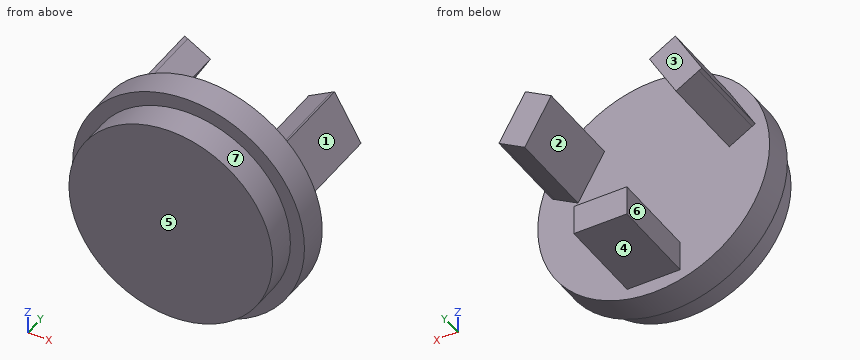
from build123d import *

# Parameters (mm, degrees)
ESQUISSE2_R        = 61.5
BOSS_EXTRU_1_DEPTH = 18
ESQUISSE3_R        = 70
BOSS_EXTRU_2_DEPTH = 18
BOSS_EXTRU_3_DEPTH = 54


with BuildPart() as part:
    # Esquisse2 → Boss.-Extru.1 (new body)
    with BuildSketch(Plane(origin=(0, 0, 0), x_dir=(1, 0, 0), z_dir=(0, 1, 0))):
        with Locations(Location((50.887518325, 23.784383565, 0), (0, 0, 270))):
            Circle(ESQUISSE2_R)
    extrude(amount=BOSS_EXTRU_1_DEPTH)

    # Esquisse3 → Boss.-Extru.2 (add)
    with BuildSketch(Plane(origin=(0, 18, 0), x_dir=(1, 0, 0), z_dir=(0, 1, 0))):
        with Locations(Location((50.887518325, 23.784383565, 0), (0, 0, 270))):
            Circle(ESQUISSE3_R)
    extrude(amount=BOSS_EXTRU_2_DEPTH)

    # Esquisse4 → Boss.-Extru.3 (add)
    with BuildSketch(Plane(origin=(0, 36, 0), x_dir=(1, 0, 0), z_dir=(0, 1, 0))):
        with BuildLine():
            ThreePointArc((-2.373044008, -6.965616435), (2.122342369, -13.688374727), (7.460993068, -19.763141096))
            Line((7.460993068, -19.763141096), (21.215413261, -11.822022896))
            Line((21.215413261, -11.822022896), (13.215413261, 2.034383565))
            Line((13.215413261, 2.034383565), (5.215413261, 15.890790026))
            Line((5.215413261, 15.890790026), (-8.539006932, 7.949671825))
            ThreePointArc((-8.539006932, 7.949671825), (-5.947430283, 0.288881513), (-2.373044008, -6.965616435))
        make_face()
        with BuildLine():
            Line((66.887518325, 67.284383565), (66.887518325, 83.166619966))
            ThreePointArc((66.887518325, 83.166619966), (58.957290978, 84.752643909), (50.887518325, 85.284383565))
            ThreePointArc((50.887518325, 85.284383565), (42.817745673, 84.752643909), (34.887518325, 83.166619966))
            Line((34.887518325, 83.166619966), (34.887518325, 67.284383565))
            Line((34.887518325, 67.284383565), (50.887518325, 67.284383565))
            Line((50.887518325, 67.284383565), (66.887518325, 67.284383565))
        make_face()
        with BuildLine():
            ThreePointArc((94.314043582, -19.763141096), (99.652694281, -13.688374727), (104.148080658, -6.965616435))
            ThreePointArc((104.148080658, -6.965616435), (107.722466934, 0.288881513), (110.314043582, 7.949671825))
            Line((110.314043582, 7.949671825), (96.55962339, 15.890790026))
            Line((96.55962339, 15.890790026), (88.55962339, 2.034383565))
            Line((88.55962339, 2.034383565), (80.55962339, -11.822022896))
            Line((80.55962339, -11.822022896), (94.314043582, -19.763141096))
        make_face()
        with BuildLine():
            ThreePointArc((110.314043582, 7.949671825), (107.722466934, 0.288881513), (104.148080658, -6.965616435))
            Line((104.148080658, -6.965616435), (112.148080658, 6.890790026))
            Line((112.148080658, 6.890790026), (110.314043582, 7.949671825))
        make_face()
        with BuildLine():
            Line((96.148080658, -20.822022896), (104.148080658, -6.965616435))
            ThreePointArc((104.148080658, -6.965616435), (99.652694281, -13.688374727), (94.314043582, -19.763141096))
            Line((94.314043582, -19.763141096), (96.148080658, -20.822022896))
        make_face()
        with BuildLine():
            ThreePointArc((50.887518325, 85.284383565), (58.957290978, 84.752643909), (66.887518325, 83.166619966))
            Line((66.887518325, 83.166619966), (66.887518325, 85.284383565))
            Line((66.887518325, 85.284383565), (50.887518325, 85.284383565))
        make_face()
        with BuildLine():
            ThreePointArc((34.887518325, 83.166619966), (42.817745673, 84.752643909), (50.887518325, 85.284383565))
            Line((50.887518325, 85.284383565), (34.887518325, 85.284383565))
            Line((34.887518325, 85.284383565), (34.887518325, 83.166619966))
        make_face()
        with BuildLine():
            Line((5.626955992, -20.822022896), (7.460993068, -19.763141096))
            ThreePointArc((7.460993068, -19.763141096), (2.122342369, -13.688374727), (-2.373044008, -6.965616435))
            Line((-2.373044008, -6.965616435), (5.626955992, -20.822022896))
        make_face()
        with BuildLine():
            Line((-10.373044008, 6.890790026), (-2.373044008, -6.965616435))
            ThreePointArc((-2.373044008, -6.965616435), (-5.947430283, 0.288881513), (-8.539006932, 7.949671825))
            Line((-8.539006932, 7.949671825), (-10.373044008, 6.890790026))
        make_face()
    extrude(amount=BOSS_EXTRU_3_DEPTH)


solid = part.part
Design review of the part built by this model. Coordinates are the model's own, in mm. Face numbers are marked on the shaded views. A direction names the side the tool comes from. Give positions to 0.01 mm unless a question says otherwise; leave off trailing zeros. Loops run counter-clockwise (first coordinate to the right, second up) from the corner with the lowest first, then second, coordinate; pieces in that order, holes last. Notation, with made-up numbers: M 80,71 L 116,71 A24 ccw 116,89 Z; hole C 25.5,53.5 d10. An arc over 180 degrees is marked long. Answer as a JSON object with one key per item and string values.
Item 1: We need section B-B (z = 14). State the section outline as (x, y) points, and give its area (3 significant figures).
Output values:
{"outline": "M -8.04,18 L 2.36,18 L 2.36,0 L 99.41,0 L 99.41,18 L 109.81,18 L 109.81,36 L 100.09,36 L 100.09,90 L 84.33,90 L 84.33,36 L 17.44,36 L 17.44,90 L 1.69,90 L 1.69,36 L -8.04,36 Z", "area": "5,570 mm2"}
Item 2: Mouldability with a two-part tool opening along X and no side actions: class the marked faces 1, 2 and 3 as pulls with the +X half, pulls with the -X half, needs draft (parallel to the pull), parting line crosses it, or undercut.
Output values:
{"face 1": "pulls with the +X half", "face 2": "undercut", "face 3": "needs draft"}
Item 3: For P1, Ø20, axis at y = 62, z = -76, coming from the -X side; P2, Ø3, axis at x = 43.5, y = 78.5, coming from the -Z side; P3, Ø1, axis at x = 102, z = -61.5, coming from the +Y side, all flat-tipped, find the tip position at first contact; note any pin that passes through.
Output values:
{"P1": "stops at x = 34.89", "P2": "stops at z = -85.28", "P3": "stops at y = 36"}
Item 4: We need section C-C (x = 29.5). State the section outline as (y, z) points.
Output values:
{"outline": "M 0,-81.45 L 18,-81.45 L 18,-90.44 L 36,-90.44 L 36,42.87 L 18,42.87 L 18,33.88 L 0,33.88 Z"}
Item 5: Wall thickness on line 1 along Y through (x, z) = (35, -84); line 2 along Y through (x, z) = (54.5, 9.5); line 3 along Z through (x, y) = (56.5, 72.5): over which ranges is each line inside the solid? List them lowest first.
Output values:
{"line 1": "y = 18 to 90", "line 2": "y = 0 to 36", "line 3": "z = -85.28 to -67.28"}
Item 6: We need section A-A (y = 56.5). State the section outline as (x, z) points, and give its area (3 significant figures).
Output values:
{"outline": "M -10.37,-6.89 L 5.22,-15.89 L 21.22,11.82 L 5.63,20.82 Z; M 34.89,-85.28 L 66.89,-85.28 L 66.89,-67.28 L 34.89,-67.28 Z; M 80.56,11.82 L 96.56,-15.89 L 112.15,-6.89 L 96.15,20.82 Z", "area": "1,730 mm2"}
Item 7: Machinability: for the marked faces 4, 5, 6 and 7, which of the approach directions +Z, -Z, +X, -X, +Y, -Y give a long, thin tool a straight path to every point of the face, cutting with its end or side? Answer none if there is none.
Output values:
{"face 4": "-Z, +X, -X, +Y", "face 5": "+Z, -Z, +X, -X, -Y", "face 6": "+Z, -Z, -X, +Y", "face 7": "-Y"}
Item 8: We need section D-D (y = 13). State the section outline as (x, z) points.
Output values:
{"outline": "C 50.89,-23.78 d123"}
